from build123d import *

# Parameters (mm, degrees)
BOSS_EXTRUDE1_DEPTH     = 18
SKETCH2_R               = 3
BOSS_EXTRUDE2_DEPTH     = 5
SKETCH2_3_R             = 3
CUT_EXTRUDE1_DEPTH      = 49.664668909
SKETCH1_3_W             = 2
SKETCH1_3_H             = 4.5
BOSS_EXTRUDE3_DEPTH     = 30
SKETCH3_OUTSIDE_W       = 56.936
SKETCH3_OUTSIDE_H       = 63.936
SKETCH3_OUTSIDE_R       = 28
CUT_EXTRUDE2_DEPTH      = 57.69435598
CUT_EXTRUDE3_START      = -18.5
CUT_EXTRUDE3_DEPTH      = 18.5
CUT_EXTRUDE4_DEPTH      = 57.587476675
CUT_EXTRUDE4_DEPTH_BACK = 10
SKETCH7_R               = 2.5
BOSS_EXTRUDE4_DEPTH     = 3
BOSS_EXTRUDE6_START     = -3
BOSS_EXTRUDE6_DEPTH     = 3
BOSS_EXTRUDE7_START     = -3
BOSS_EXTRUDE7_DEPTH     = 3
BOSS_EXTRUDE8_START     = -3
BOSS_EXTRUDE8_DEPTH     = 3
CUT_EXTRUDE5_DEPTH      = 43.804159814
CUT_EXTRUDE5_DEPTH_BACK = 43.804159814
SKETCH7_3_R             = 2.5


# Read off the part's stored shape, not the designer's step: Cut-Extrude3
with BuildPart() as part:
    # Sketch1 → Boss-Extrude1 (new body)
    with BuildSketch(Plane(origin=(0, 0, 0), x_dir=(1, 0, 0), z_dir=(0, 1, 0))):
        Polygon((7.5, 3), (-3, 3), (-3, -7), (5.5, -7), (5.5, -11.5), (1.5, -11.5), (1.5, -15.5), (33.5, -15.5), (33.5, -11.5), (29.5, -11.5), (29.5, -7), (38, -7), (38, 3), (27.5, 3), (27.5, 9), (7.5, 9), align=None)
        Polygon((24.5, 0), (35, 0), (35, -4), (24.5, -4), (24.5, -10), (10.5, -10), (10.5, -4), (0, -4), (0, 0), (10.5, 0), (10.5, 6), (24.5, 6), align=None, mode=Mode.SUBTRACT)
    extrude(amount=BOSS_EXTRUDE1_DEPTH)

    # Sketch2 → Boss-Extrude2 (add)
    with BuildSketch(Plane(origin=(0, 0, -9), x_dir=(-1, 0, 0), z_dir=(0, 0, -1))):
        with BuildLine():
            ThreePointArc((-20.81662479, 18), (-20.337274331, 7.713235926), (-11.5, 13))
            ThreePointArc((-11.5, 13), (-12.213235926, 15.837274331), (-14.18337521, 18))
            Line((-14.18337521, 18), (-20.81662479, 18))
        make_face()
        with Locations((-17.5, 13)):
            Circle(SKETCH2_R, mode=Mode.SUBTRACT)
    extrude(amount=BOSS_EXTRUDE2_DEPTH)

    # Sketch2<3> → Cut-Extrude1 (cut, through all)
    with BuildSketch(Plane(origin=(0, 0, -9), x_dir=(-1, 0, 0), z_dir=(0, 0, -1))):
        with Locations((-17.5, 13)):
            Circle(SKETCH2_3_R)
    extrude(amount=-CUT_EXTRUDE1_DEPTH, mode=Mode.SUBTRACT)

    # Sketch1<3> → Boss-Extrude3 (add)
    with BuildSketch(Plane(origin=(0, 0, 0), x_dir=(1, 0, 0), z_dir=(0, 1, 0))):
        Polygon((0, -4), (0, 0), (0, 3), (-3, 3), (-3, -7), (5.5, -7), (7.5, -7), (7.5, -11.5), (7.5, -13), (27.5, -13), (27.5, -11.5), (27.5, -7), (29.5, -7), (38, -7), (38, 3), (35, 3), (35, 0), (35, -4), (24.5, -4), (24.5, -10), (10.5, -10), (10.5, -4), align=None)
        with Locations((28.5, -9.25)):
            Rectangle(SKETCH1_3_W, SKETCH1_3_H)
        Polygon((7.5, -11.5), (5.5, -11.5), (1.5, -11.5), (1.5, -15.5), (33.5, -15.5), (33.5, -11.5), (29.5, -11.5), (27.5, -11.5), (27.5, -13), (7.5, -13), align=None)
        with Locations((6.5, -9.25)):
            Rectangle(SKETCH1_3_W, SKETCH1_3_H)
    extrude(amount=-BOSS_EXTRUDE3_DEPTH)

    # Sketch3 outside → Cut-Extrude2 (cut, through all)
    with BuildSketch(Plane.XY.offset(15.5)):
        with Locations((17.5, -6)):
            Rectangle(SKETCH3_OUTSIDE_W, SKETCH3_OUTSIDE_H)
        with Locations((17.5, -1.797525342)):
            Circle(SKETCH3_OUTSIDE_R, mode=Mode.SUBTRACT)
    extrude(amount=-CUT_EXTRUDE2_DEPTH, mode=Mode.SUBTRACT)

    # Cut-Extrude3 outline → Cut-Extrude3 (cut)
    with BuildSketch(Plane.XY.offset(15.5).offset(CUT_EXTRUDE3_START)):
        with BuildLine():
            Line((32.171400751, 18), (38, 0.89725692))
            Line((38, 0.89725692), (38, 17.274705781))
            ThreePointArc((38, 17.274705781), (37.653490195, 17.640500097), (37.300454296, 18))
            Line((37.300454296, 18), (32.171400751, 18))
        make_face()
        with BuildLine():
            Line((2.828599249, 18), (-2.300454296, 18))
            ThreePointArc((-2.300454296, 18), (-2.653490195, 17.640500097), (-3, 17.274705781))
            Line((-3, 17.274705781), (-3, 0.89725692))
            Line((-3, 0.89725692), (2.828599249, 18))
        make_face()
    extrude(amount=CUT_EXTRUDE3_DEPTH, mode=Mode.SUBTRACT)

    # Sketch5 → Cut-Extrude4 (cut, two sides: drawn at the far end of the back side and taken through both)
    with BuildSketch(Plane.XY.offset(15.5).offset(-CUT_EXTRUDE4_DEPTH_BACK)):
        with BuildLine():
            ThreePointArc((10.5, -28.908408765), (17.5, -29.797525342), (24.5, -28.908408765))
            Line((24.5, -28.908408765), (24.5, -15.797525342))
            ThreePointArc((24.5, -15.797525342), (23.035533906, -12.261991436), (19.5, -10.797525342))
            Line((19.5, -10.797525342), (15.5, -10.797525342))
            ThreePointArc((15.5, -10.797525342), (11.964466094, -12.261991436), (10.5, -15.797525342))
            Line((10.5, -15.797525342), (10.5, -28.908408765))
        make_face()
    extrude(amount=CUT_EXTRUDE4_DEPTH + CUT_EXTRUDE4_DEPTH_BACK, mode=Mode.SUBTRACT)

    # Sketch7 → Boss-Extrude4 (add)
    # profile 1 of 2: a face of its own
    with BuildSketch(Plane.ZY.offset(-24.5)):
        with BuildLine():
            Line((-5, -15), (4, -15))
            Line((4, -15), (4, -3))
            Line((4, -3), (-5, -3))
            ThreePointArc((-5, -3), (-7.121320344, -3.878679656), (-8, -6))
            Line((-8, -6), (-8, -12))
            ThreePointArc((-8, -12), (-7.121320344, -14.121320344), (-5, -15))
        make_face()
        with Locations((-2, -9)):
            Circle(SKETCH7_R, mode=Mode.SUBTRACT)
    # profile 2 of 2: a face of its own
    with BuildSketch(Plane.ZY.offset(-24.5)):
        with Locations((-2, -9)):
            Circle(SKETCH7_R)
    extrude(amount=-BOSS_EXTRUDE4_DEPTH)

    # Sketch9 → Boss-Extrude6 (add)
    with BuildSketch(Plane(origin=(10.5, 0, 0), x_dir=(0, 0, -1), z_dir=(1, 0, 0)).offset(BOSS_EXTRUDE6_START)):
        with BuildLine():
            Line((-4, -15), (5, -15))
            ThreePointArc((5, -15), (7.121320344, -14.121320344), (8, -12))
            Line((8, -12), (8, -6))
            ThreePointArc((8, -6), (7.121320344, -3.878679656), (5, -3))
            Line((5, -3), (-4, -3))
            Line((-4, -3), (-4, -15))
        make_face()
    extrude(amount=BOSS_EXTRUDE6_DEPTH)

    # Sketch10 → Boss-Extrude7 (add)
    with BuildSketch(Plane.ZY.offset(-35).offset(BOSS_EXTRUDE7_START)):
        with BuildLine():
            Line((-5, -15), (-3, -15))
            Line((-3, -15), (-3, -3))
            Line((-3, -3), (-5, -3))
            ThreePointArc((-5, -3), (-7.121320344, -3.878679656), (-8, -6))
            Line((-8, -6), (-8, -12))
            ThreePointArc((-8, -12), (-7.121320344, -14.121320344), (-5, -15))
        make_face()
    extrude(amount=BOSS_EXTRUDE7_DEPTH)

    # Sketch11 → Boss-Extrude8 (add)
    with BuildSketch(Plane(origin=(0, 0, 0), x_dir=(0, 0, -1), z_dir=(1, 0, 0)).offset(BOSS_EXTRUDE8_START)):
        with BuildLine():
            Line((5, -3), (3, -3))
            Line((3, -3), (3, -6.708712153))
            ThreePointArc((3, -6.708712153), (4.091650066, -7.630693606), (4.5, -9))
            ThreePointArc((4.5, -9), (4.091650066, -10.369306394), (3, -11.291287847))
            Line((3, -11.291287847), (3, -15))
            Line((3, -15), (5, -15))
            ThreePointArc((5, -15), (7.121320344, -14.121320344), (8, -12))
            Line((8, -12), (8, -6))
            ThreePointArc((8, -6), (7.121320344, -3.878679656), (5, -3))
        make_face()
        with BuildLine():
            ThreePointArc((4.5, -9), (4.091650066, -7.630693606), (3, -6.708712153))
            Line((3, -6.708712153), (3, -11.291287847))
            ThreePointArc((3, -11.291287847), (4.091650066, -10.369306394), (4.5, -9))
        make_face()
        with BuildLine():
            Line((3, -11.291287847), (3, -6.708712153))
            ThreePointArc((3, -6.708712153), (-0.5, -9), (3, -11.291287847))
        make_face()
    extrude(amount=BOSS_EXTRUDE8_DEPTH)

    # Sketch7<3> → Cut-Extrude5 (cut, two sides: drawn at the far end of the back side and taken through both)
    with BuildSketch(Plane.ZY.offset(-24.5).offset(-CUT_EXTRUDE5_DEPTH_BACK)):
        with Locations((-2, -9)):
            Circle(SKETCH7_3_R)
    extrude(amount=CUT_EXTRUDE5_DEPTH + CUT_EXTRUDE5_DEPTH_BACK, mode=Mode.SUBTRACT)


solid = part.part
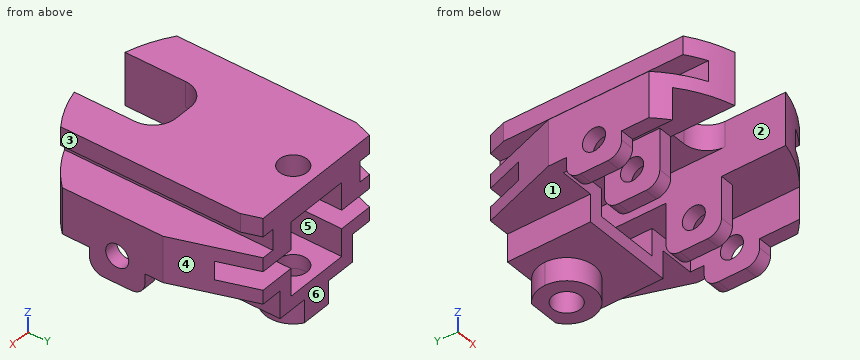
Work out the finished part from the listing and answer in its coordinate system (mm). Face numbers are marked on the shaded views. A direction names the side the tool comes from. Give positions to 0.01 mm unless a question says otherwise; leave off trailing zeros. Write each loop counter-clockwise with the first axis right and the second up, starting at its lowest first coordinate (ties: lowest second). Pieces come first, ordered by that corner, then holes. Notation, with made-up numbers: M 41,-14 L 86,-14 A15 ccw 86,12 Z; hole C 21,49 d3. An arc over 180 degrees is marked long. Answer as CSV lines item,"result".
Q1. The mould has two halves that part along X. Classify the marked faces 4, 5 and 6: +X half, -X half, draft (parallel to the pull), parting line (faces both ways), or undercut.
A:
face 4,"+X half"
face 5,"undercut"
face 6,"draft"
Q2. A tool of negligible diameter and unlimited length cuts with its end or side. For the marked faces 1, 2 and 3, from which of +Z, -Z, +X, -X, +Y, -Y can it reach the whole face along a straight path? Write none if from no direction.
A:
face 1,"-Z, -X, +Y"
face 2,"-Y"
face 3,"+Z, +X, +Y, -Y"
Q3. Find the intervals of material crossed by probe 1 along X at (y, z) = (-13, -1); probe 2 along Y at (x, z) = (26.05, -2); probe 3 along Z at (x, y) = (32, 3.5), in increasing order. Write a range as [from, to].
A:
probe 1,"x = [-3, 0], [7.5, 10.5], [24.5, 27.5], [35, 38]"
probe 2,"y = [-15, -11.5], [-6.5, -3], [0, 18]"
probe 3,"z = [-3, 0], [4, 7], [11.5, 15.5]"
Q4. A cutting plane is placed at B-B on x = 8.5. Write down the section's boundary in (y, z), plus the area to 3 significant figures.
A:
outline,"M -28.31,4 L -15,4 L -15,-5 A3 ccw -12,-8 L -6,-8 A3 ccw -3,-5 L -3,4 L 18,4 L 18,15.5 L -28.31,15.5 Z; M 0,-9 L 18,-9 L 18,0 L 0,0 Z; hole C -9,-2 d5"
area,"815 mm²"
Q5. A cutting plane is placed at A-A on z = 6. Write down the section's boundary in (x, y), plus the area to 3 significant figures.
A:
outline,"M -3,-20.87 A28 ccw 10.5,-28.91 L 10.5,18 L 2.83,18 L -3,0.9 Z; M 24.5,-28.91 A28 ccw 38,-20.87 L 38,0.9 L 32.17,18 L 24.5,18 Z"
area,"1,080 mm²"
Q6. Given P1, Ø15.5, axis at x = 16.5, y = -2, coming from the -Z side; P2, Ø2.5, axis at x = 37, y = -8, coming from the -Z side; P3, Ø6, axis at y = -11, z = -2.5, coming from the +X side; P4, Ø2, axis at x = 31.5, y = -5, coming from the -Z side, each flat-ended and moving along its own axis, determine where each tip first touches the part or whether it passes through.
A:
P1,"stops at z = -9"
P2,"stops at z = -8"
P3,"stops at x = 38"
P4,"stops at z = 4"
Q7. A cutting plane is placed at C-C on y = -22. Write down the section's boundary in (x, z), plus the area to 3 significant figures.
A:
outline,"M -1.89,-3 L 0,-3 L 0,4 L 10.5,4 L 10.5,15.5 L 1.5,15.5 L 1.5,11.5 L 5.5,11.5 L 5.5,7 L -1.89,7 Z; M 24.5,4 L 35,4 L 35,-3 L 36.89,-3 L 36.89,7 L 29.5,7 L 29.5,11.5 L 33.5,11.5 L 33.5,15.5 L 24.5,15.5 Z"
area,"218 mm²"
